Part model, mm, in its own coordinate system. Face numbers are marked on the shaded views. A direction names the side the tool comes from. Round coordinates to 2 decimals unless told otherwise and drop trailing zeros. Loops run counter-clockwise (first coordinate to the right, second up) from the corner with the lowest first, then second, coordinate; pieces in that order, holes last. Notation, with made-up numbers: (5.25, 40) - (57.25, 40) arc R18 ccw to (57.25, 52) - close; hole circle Ø1 at (43, 69). An arc over 180 degrees is marked (long way). Write each question's results on one line, items separated by ' | '. Start each with the question number.
(1) Cut at A-A, the plane x = 0. List the corners of the cut face in (y, z).
(2) Mould opens along Y. For the marked faces 1, 2 and 3 say: released by +Y, released by -Y, zero draft, split by the parting line, or undercut.
(3) Cut at B-B, the plane z = 5.5. List the corners of the cut face in (x, y).
(4) Tool access for the marked faces 4, 5, 6, 7 and 8: list every direction of +Z, -Z, +X, -X, +Y, -Y with a clear straight run to the whole face (end or side of a thin tool).
(5) Drill centre lines: L1, parallel to Y at x = 0, z = 3.3; L2, parallel to Y at x = 0, z = 2.45. Where is each one in solid material? Low to high.
(6) Flat gauge pins, fed straight in: P1, Ø0.6, axis at x = 0, z = 4, coming from the +Y side; P2, Ø4, axis at x = 0, y = 0, coming from the -Z side; P3, Ø1.3, axis at x = 0, y = 0, coming from the -Z side. Where does each tip first touch, or does it go through?
from build123d import *

# Parameters (mm, degrees)
F1_DEPTH = 8
F2_R     = 1
F3_DEPTH = 5
F4_DEPTH = 3


with BuildPart() as f1:
    # F0 (on Top) → F1 (new body)
    with BuildSketch(Plane.XY):
        Polygon((-11.6672618896, 17.3241161391), (-17.3241161391, 11.6672618896), (-5.6568542495, 0), (-17.3241161391, -11.6672618896), (-11.6672618896, -17.3241161391), (0, -5.6568542495), (11.6672618896, -17.3241161391), (17.3241161391, -11.6672618896), (5.6568542495, 0), (17.3241161391, 11.6672618896), (11.6672618896, 17.3241161391), (0, 5.6568542495), align=None)
        with BuildLine():
            ThreePointArc((-1.7349351573, -1.8), (-0.9779218033, 2.3007974588), (2.5, 0))
            ThreePointArc((2.5, 0), (2.3007974588, -0.9779218033), (1.7349351573, -1.8))
            ThreePointArc((1.7349351573, -1.8), (0, -2.5), (-1.7349351573, -1.8))
        make_face(mode=Mode.SUBTRACT)
        with BuildLine():
            Line((1.7349351573, -1.8), (-1.7349351573, -1.8))
            ThreePointArc((-1.7349351573, -1.8), (0, -2.5), (1.7349351573, -1.8))
        make_face()
        with BuildLine():
            ThreePointArc((1.7349351573, -1.8), (2.3007974588, -0.9779218033), (2.5, 0))
            ThreePointArc((2.5, 0), (-0.9779218033, 2.3007974588), (-1.7349351573, -1.8))
            Line((-1.7349351573, -1.8), (1.7349351573, -1.8))
        make_face()
    extrude(amount=F1_DEPTH)

    # F2
    f2_edges = [f1.edges().sort_by_distance(p)[0] for p in [
        (-14.495689, 14.495689, 8),
        (-11.490485, 5.833631, 8),
        (-11.490485, -5.833631, 8),
        (-14.495689, -14.495689, 8),
        (-5.833631, -11.490485, 8),
        (5.833631, -11.490485, 8),
        (14.495689, -14.495689, 8),
        (11.490485, -5.833631, 8),
        (11.490485, 5.833631, 8),
        (14.495689, 14.495689, 8),
        (5.833631, 11.490485, 8),
        (-5.833631, 11.490485, 8),
        (-11.667262, -17.324116, 4),
        (-17.324116, -11.667262, 4),
        (-17.324116, 11.667262, 4),
        (11.667262, -17.324116, 4),
        (17.324116, -11.667262, 4),
        (17.324116, 11.667262, 4),
        (11.667262, 17.324116, 4),
        (-11.667262, 17.324116, 4),
        (0, 5.656854, 4),
        (-5.656854, 0, 4),
        (0, -5.656854, 4),
        (5.656854, 0, 4),
    ]]
    fillet(f2_edges, radius=F2_R)

    # F0 (on Top) → F3 (cut)
    with BuildSketch(Plane.XY):
        with BuildLine():
            ThreePointArc((1.7349351573, -1.8), (2.3007974588, -0.9779218033), (2.5, 0))
            ThreePointArc((2.5, 0), (-0.9779218033, 2.3007974588), (-1.7349351573, -1.8))
            Line((-1.7349351573, -1.8), (1.7349351573, -1.8))
        make_face()
    extrude(amount=F3_DEPTH, mode=Mode.SUBTRACT)

    # F0 (on Top) → F4 (cut)
    with BuildSketch(Plane.XY):
        with BuildLine():
            Line((1.7349351573, -1.8), (-1.7349351573, -1.8))
            ThreePointArc((-1.7349351573, -1.8), (0, -2.5), (1.7349351573, -1.8))
        make_face()
    extrude(amount=F4_DEPTH, mode=Mode.SUBTRACT)


solid = f1.part
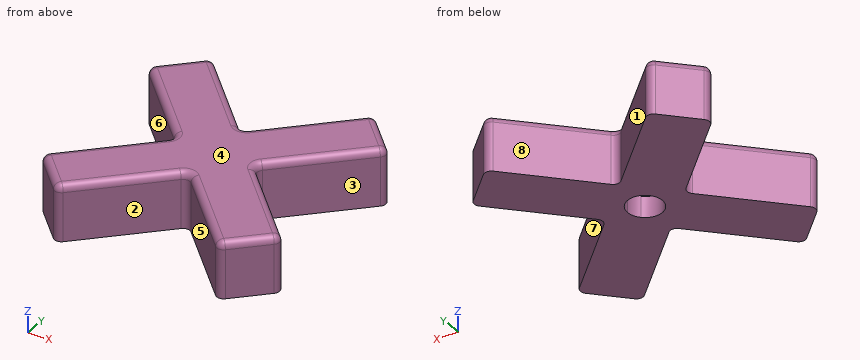
A:
1) outline: (-6.07, 0) - (-2.5, 0) - (-2.5, 3) - (-1.8, 3) - (-1.8, 5) - (2.5, 5) - (2.5, 0) - (6.07, 0) - (6.07, 7) arc R1 ccw to (5.07, 8) - (-5.07, 8) arc R1 ccw to (-6.07, 7) - close
2) face 1: released by +Y | face 2: released by -Y | face 3: undercut
3) outline: (-16.62, -12.37) - (-12.37, -16.62) arc R1 ccw to (-10.96, -16.62) - (-0.71, -6.36) arc R1 cw to (0.71, -6.36) - (10.96, -16.62) arc R1 ccw to (12.37, -16.62) - (16.62, -12.37) arc R1 ccw to (16.62, -10.96) - (6.36, -0.71) arc R1 cw to (6.36, 0.71) - (16.62, 10.96) arc R1 ccw to (16.62, 12.37) - (12.37, 16.62) arc R1 ccw to (10.96, 16.62) - (0.71, 6.36) arc R1 cw to (-0.71, 6.36) - (-10.96, 16.62) arc R1 ccw to (-12.37, 16.62) - (-16.62, 12.37) arc R1 ccw to (-16.62, 10.96) - (-6.36, 0.71) arc R1 cw to (-6.36, -0.71) - (-16.62, -10.96) arc R1 ccw to start
4) face 4: +Z, +X, -X, +Y, -Y | face 5: +Z, -Z, -Y | face 6: +Z, -Z, -X | face 7: +Z, -Z, +X | face 8: +Z, -Z, +Y
5) L1: -6.07 to -1.8, 2.5 to 6.07 | L2: -6.07 to -2.5, 2.5 to 6.07
6) P1: y = 6.12 | P2: z = 3 | P3: z = 5
